Design review of the part built by this model. Coordinates are the model's own, in mm. Face numbers are marked on the shaded views. A direction names the side the tool comes from. Coordinates: 2 decimals unless noted, no trailing zeros. Loops run counter-clockwise (first coordinate to the right, second up) from the corner with the lowest first, then second, coordinate; pieces in that order, holes last. Notation, with made-up numbers: M -25,70.25 L 20,70.25 A8 ccw 20,85.25 Z; hole C 0.25,-4.75 d10. An arc over 180 degrees is marked long. Put each result on its own line as item: value. Start each with the question number.
(1) Take a section at D-D, the plane z = 7.5. Give the boundary of the cut face in (x, y), then the cut area to 3 significant figures.
(2) Clearance check with flat-ended pins moving along their axes: pin 1 (6 mm diameter, centred on x = -6, y = 6.5, fed in from -Z); pin 2 (10 mm diameter, centred on x = 19, y = 21, fed in from -Z); pin 3 (6 mm diameter, centred on y = 21, z = 14, fed in from -X). State where each tip first meets the part, or that it passes through.
(3) For probe 1 along Z at (x, y) = (15.5, 9.75) (3 decimals); probe 2 along Z at (x, y) = (2, 25.25), list the stretches that pass through material, from the lowest coordinate up. Write a range as [from, to].
(4) Take a section at C-C, the plane x = -15.5. Give the boundary of the cut face in (y, z) (3 decimals), then the cut area to 3 significant figures.
(5) Take a section at B-B, the plane z = -15.5. Give the boundary of the cut face in (x, y) (3 decimals), then the cut area to 3 significant figures.
(6) The part is to be moulded in two halves that separate along X. For the marked faces 3, 4 and 5, say which applies: +X half, -X half, draft (parallel to the pull), parting line (faces both ways), or undercut.
(7) Take a section at A-A, the plane y = 11.5. Give the boundary of the cut face in (x, z) (3 decimals).
(8) For the marked faces 1 and 2, list the 3-axis set-ups (+Z, -Z, +X, -X, +Y, -Y) from which the entire face can be reached by the end or side of a thin tool; tool diameter is ignored.
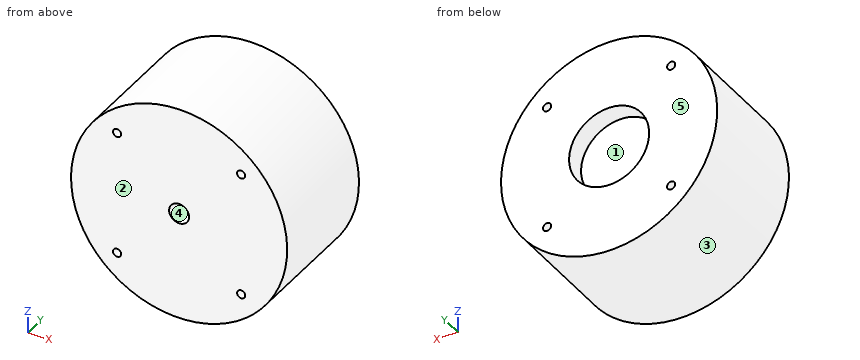
```python
from build123d import *

# Parameters (mm, degrees)
SKETCH_1_R           = 27
EXTRUDE_1_DEPTH      = 30
HOLE_WIZARD_M2_5_1_D = 2.05
SKETCH_7_R           = 2.5
CUT_EXTRUDE_1_DEPTH  = 24
SKETCH_8_R           = 10
CUT_EXTRUDE_2_DEPTH  = 5


with BuildPart() as part:
    # 草图1 → 凸台-拉伸1 (new body)
    with BuildSketch(Plane(origin=(0, 0, 0), x_dir=(1, 0, 0), z_dir=(0, 1, 0))):
        with Locations(Location((0, 0, 0), (0, 0, 270))):
            Circle(SKETCH_1_R)
    extrude(amount=EXTRUDE_1_DEPTH)

    # M2.5 螺纹孔1 (through all)
    with Locations(Plane(origin=(0, 0, 0), x_dir=(-1, 0, 0), z_dir=(0, -1, 0))):
        with Locations((15.5, 15.5), (-15.5, 15.5), (-15.5, -15.5), (15.5, -15.5)):
            Hole(HOLE_WIZARD_M2_5_1_D / 2)

    # 草图7 → 切除-拉伸1 (cut)
    with BuildSketch(Plane.XZ):
        with Locations(Location((0, 0, 0), (0, 0, 270))):
            Circle(SKETCH_7_R)
    extrude(amount=-CUT_EXTRUDE_1_DEPTH, mode=Mode.SUBTRACT)

    # 草图8 → 切除-拉伸2 (cut)
    with BuildSketch(Plane(origin=(0, 30, 0), x_dir=(1, 0, 0), z_dir=(0, 1, 0))):
        with Locations(Location((0, 0, 0), (0, 0, 270))):
            Circle(SKETCH_8_R)
    extrude(amount=-CUT_EXTRUDE_2_DEPTH, mode=Mode.SUBTRACT)


solid = part.part
```
Computed values:
1. outline: M -25.94,0 L 25.94,0 L 25.94,30 L 6.61,30 L 6.61,25 L -6.61,25 L -6.61,30 L -25.94,30 Z
1. area: 1,490 mm^2
2. pin 1: stops at z = -26.83
2. pin 2: stops at z = -23.09
2. pin 3: stops at x = -24.66
3. probe 1: z = [-22.108, -16.525], [-14.475, 14.475], [16.525, 22.108]
3. probe 2: z = [-26.93, -9.8], [9.8, 26.93]
4. outline: M 0,-22.108 L 30,-22.108 L 30,-16.525 L 0,-16.525 Z; M 0,-14.475 L 30,-14.475 L 30,14.475 L 0,14.475 Z; M 0,16.525 L 30,16.525 L 30,22.108 L 0,22.108 Z
4. area: 1,200 mm^2
5. outline: M -22.108,0 L -16.525,0 L -16.525,30 L -22.108,30 Z; M -14.475,0 L 14.475,0 L 14.475,30 L -14.475,30 Z; M 16.525,0 L 22.108,0 L 22.108,30 L 16.525,30 Z
5. area: 1,200 mm^2
6. face 3: parting line
6. face 4: undercut
6. face 5: draft
7. outline: C 0,0 d54; hole C -15.5,-15.5 d2.05; hole C -15.5,15.5 d2.05; hole C 0,0 d5; hole C 15.5,-15.5 d2.05; hole C 15.5,15.5 d2.05
8. face 1: +Y
8. face 2: +Z, -Z, +X, -X, -Y
